from build123d import *

# Parameters (mm, degrees)
ESQUISSE1_R                 = 35
ESQUISSE1_R_2               = 10
BOSS_EXTRU_1_DEPTH          = 7.5
ESQUISSE2_R                 = 32.5
ESQUISSE2_R_2               = 10
BOSS_EXTRU_2_DEPTH          = 20
ESQUISSE3_R                 = 35
ESQUISSE3_R_2               = 10
BOSS_EXTRU_3_DEPTH          = 5
ESQUISSE4_R                 = 32.5
ESQUISSE4_R_2               = 10
BOSS_EXTRU_4_DEPTH          = 20
ESQUISSE5_R                 = 35
ESQUISSE5_R_2               = 10
BOSS_EXTRU_5_DEPTH          = 7.5
ESQUISSE7_W                 = 0.6
ESQUISSE7_H                 = 2.216048933
ENL_V_MAT_EXTRU_3_DEPTH     = 7.5
ENL_V_MAT_EXTRU_6_OUTLINE_W = 5
ENL_V_MAT_EXTRU_6_OUTLINE_H = 4.514677359
ENL_V_START                 = 9.580417676
ENL_V_MAT_EXTRU_7_OUTLINE_R = 2.5
ENL_V_MAT_EXTRU_7_DEPTH     = 18.40495848


# Read off the part's stored shape, not the designer's step: Enlèv. mat.-Extru.6, Enlèv. mat.-Extru.7
with BuildPart() as part:
    # Esquisse1 → Boss.-Extru.1 (new body)
    with BuildSketch(Plane.XY):
        Circle(ESQUISSE1_R)
        Circle(ESQUISSE1_R_2, mode=Mode.SUBTRACT)
    extrude(amount=BOSS_EXTRU_1_DEPTH)

    # Esquisse2 → Boss.-Extru.2 (add)
    with BuildSketch(Plane.XY.offset(7.5)):
        Circle(ESQUISSE2_R)
        Circle(ESQUISSE2_R_2, mode=Mode.SUBTRACT)
    extrude(amount=BOSS_EXTRU_2_DEPTH)

    # Esquisse3 → Boss.-Extru.3 (add)
    with BuildSketch(Plane.XY.offset(27.5)):
        Circle(ESQUISSE3_R)
        Circle(ESQUISSE3_R_2, mode=Mode.SUBTRACT)
    extrude(amount=BOSS_EXTRU_3_DEPTH)

    # Esquisse4 → Boss.-Extru.4 (add)
    with BuildSketch(Plane.XY.offset(32.5)):
        Circle(ESQUISSE4_R)
        Circle(ESQUISSE4_R_2, mode=Mode.SUBTRACT)
    extrude(amount=BOSS_EXTRU_4_DEPTH)

    # Esquisse5 → Boss.-Extru.5 (add)
    with BuildSketch(Plane.XY.offset(52.5)):
        Circle(ESQUISSE5_R)
        Circle(ESQUISSE5_R_2, mode=Mode.SUBTRACT)
    extrude(amount=BOSS_EXTRU_5_DEPTH)

    # Esquisse7 → Enlèv. mat.-Extru.3 (cut)
    with BuildSketch(Plane(origin=(0, 0, 0), x_dir=(-1, 0, 0), z_dir=(0, 0, -1))):
        with Locations((0, 35.093400622)):
            Rectangle(ESQUISSE7_W, ESQUISSE7_H)
    extrude(amount=-ENL_V_MAT_EXTRU_3_DEPTH, mode=Mode.SUBTRACT)

    # Enlèv. mat.-Extru.6 outline → Enlèv. mat.-Extru.6 (revolve, cut)
    with BuildSketch(Plane(origin=(0.366285961, 0, 15), x_dir=(1, 0, 0), z_dir=(0, 0, 1))):
        with Locations((2.5, 30.242714836)):
            Rectangle(ENL_V_MAT_EXTRU_6_OUTLINE_W, ENL_V_MAT_EXTRU_6_OUTLINE_H)
    revolve(axis=Axis((0.366285961, 0, 15), (0, 1, 0)), mode=Mode.SUBTRACT)

    # Enlèv. mat.-Extru.7 outline → Enlèv. mat.-Extru.7 (cut)
    with BuildSketch(Plane(origin=(0, 0, 0), x_dir=(1, 0, 0), z_dir=(0, 1, 0)).offset(ENL_V_START)):
        with Locations((0.366285961, -15)):
            Circle(ENL_V_MAT_EXTRU_7_OUTLINE_R)
    extrude(amount=ENL_V_MAT_EXTRU_7_DEPTH, mode=Mode.SUBTRACT)


solid = part.part
Geometry: final body of the model. Coordinates: model frame, mm. A direction names the side the tool comes from. Give positions to 0.01 mm unless a question says otherwise; leave off trailing zeros. Write each loop counter-clockwise with the first axis right and the second up, starting at its lowest first coordinate (ties: lowest second). Pieces come first, ordered by that corner, then holes. Notation, with made-up numbers: (87.5, 45.5) -> (120.5, 45.5) arc R27 ccw to (120.5, 68.5) -> close; hole circle Ø11 at (84.25, -17.5). An arc over 180 degrees is marked (long way). Answer as a JSON object with one key per item and string values.
1. Ray query, probe 1 along Y at (x, z) = (-0.5, 20); probe 2 along Y at (x, z) = (-5.5, 39); probe 3 along X at (y, z) = (13.5, 15). Return the intervals inside material, ascending. Write a range as from..to.
Ans:
{"probe 1": "y = -32.5..-9.99, 9.99..32.5", "probe 2": "y = -32.03..-8.35, 8.35..32.03", "probe 3": "x = -29.56..-2.13, 2.87..29.56"}
2. Mould query, pull axis X, two halves, no side actions, for faces 1 (the cylindrical face through (-7.045, -31.727, 17.36)), 2 (the flat face through (3, 27.985, 16)), 3 (the flat face through (23.2, -23.2, 32.5)). Classes: pulls with the +X half, pulls with the -X half, needs draft (parallel to the pull), parting line crosses it, or undercut.
Ans:
{"face 1": "parting line crosses it", "face 2": "undercut", "face 3": "needs draft"}
3. Cut plane B-B on z = 31. Output: boundary loops of the cut face in (x, y).
Ans:
{"outline": "circle Ø70 at (0, 0); hole circle Ø20 at (0, 0)"}
4. Access query for faces 4 (the cylindrical face through (-28, -21, 56)), 5 (the cylindrical face through (31, 9.76, 42.36)), 6 (the cylindrical face through (-0.18, 18.65, 17.44)). Directions: +Z, -Z, +X, -X, +Y, -Y. A direction counts if a zero-diameter tool reaches every point of the face in a straight line with its end or side. Return the directions, or none.
Ans:
{"face 4": "+Z, -Z", "face 5": "none", "face 6": "+Y"}
5. Contact query for flat-ended pins moving along their axis: pin 1 (1.5 mm diameter, centred on x = -15.5, z = 52.5, fed in from -Y); pin 2 (3 mm diameter, centred on y = 17, z = 43, fed in from -X); pin 3 (6 mm diameter, centred on y = 26.5, z = 39.5, fed in from +X). Output: stop coordinate, or through.
Ans:
{"pin 1": "stops at y = -31.74", "pin 2": "stops at x = -28.57", "pin 3": "stops at x = 22.45"}
6. Cut plane A-A on y = 27. Output: boundary loops of the cut face in (x, z).
Ans:
{"outline": "(-22.27, 0) -> (22.27, 0) -> (22.27, 7.5) -> (18.09, 7.5) -> (18.09, 27.5) -> (22.27, 27.5) -> (22.27, 32.5) -> (18.09, 32.5) -> (18.09, 52.5) -> (22.27, 52.5) -> (22.27, 60) -> (-22.27, 60) -> (-22.27, 52.5) -> (-18.09, 52.5) -> (-18.09, 32.5) -> (-22.27, 32.5) -> (-22.27, 27.5) -> (-18.09, 27.5) -> (-18.09, 7.5) -> (-22.27, 7.5) -> close; hole circle Ø5 at (0.37, 15)"}
7. Cut plane D-D on y = -29. Output: boundary loops of the cut face in (x, z), and give its area (3 significant figures).
Ans:
{"outline": "(-19.6, 0) -> (19.6, 0) -> (19.6, 7.5) -> (14.67, 7.5) -> (14.67, 27.5) -> (19.6, 27.5) -> (19.6, 32.5) -> (14.67, 32.5) -> (14.67, 52.5) -> (19.6, 52.5) -> (19.6, 60) -> (-19.6, 60) -> (-19.6, 52.5) -> (-14.67, 52.5) -> (-14.67, 32.5) -> (-19.6, 32.5) -> (-19.6, 27.5) -> (-14.67, 27.5) -> (-14.67, 7.5) -> (-19.6, 7.5) -> close", "area": "1,960 mm^2"}
8. Cut plane C-C on x = 14. Output: boundary loops of the cut face in (y, z), and give its area (3 significant figures).
Ans:
{"outline": "(-32.08, 0) -> (32.08, 0) -> (32.08, 7.5) -> (29.33, 7.5) -> (29.33, 27.5) -> (32.08, 27.5) -> (32.08, 32.5) -> (29.33, 32.5) -> (29.33, 52.5) -> (32.08, 52.5) -> (32.08, 60) -> (-32.08, 60) -> (-32.08, 52.5) -> (-29.33, 52.5) -> (-29.33, 32.5) -> (-32.08, 32.5) -> (-32.08, 27.5) -> (-29.33, 27.5) -> (-29.33, 7.5) -> (-32.08, 7.5) -> close", "area": "3,630 mm^2"}
